Verification items for the finished model (mm, model axes). Coordinates: 2 decimals unless noted, no trailing zeros. Order: outer loops, then holes, each group sorted by start corner. A loop starts at its lowest first (then second) coordinate and runs counter-clockwise, first axis right, second up. Notation, with made-up numbers: M 36,-17.75 L 93,-17.75 A19 cw 93,10.25 Z; hole C 47,78 d8. An arc over 180 degrees is marked long. Return JSON: item names as keys, results as strings. Group by question number.
1. Material ranges on line 1 along Y through (x, z) = (27, 0.95); line 2 along X through (y, z) = (24.5, 1.35); line 3 along X through (y, z) = (26.5, 0.65), recorded low to high.
2. Section check C-C, the plane z = 1.95. Record the cut outline in (x, y), plus the area to 3 significant figures.
3. Mould release check, pull along X, two halves, no side actions. Record for faces 1 (the flat face through (44, 38, 0)), 2 (the cylindrical face through (55.532, 65.783, 1.479)), 3 (the flat face through (56, 34.748, 1)): +X half, -X half, draft (parallel to the pull), parting line (faces both ways), or undercut.
4. Gauge pin test, flat ends, axial feed: pin 1 (1.5 mm diameter, centred on x = 59, z = 2, fed in from +Y); pin 2 (1.5 mm diameter, centred on x = 55, z = 0.5, fed in from -Y); pin 3 (1.5 mm diameter, centred on x = 54, z = 1, fed in from -Y); pin 4 (1 mm diameter, centred on x = 15.5, y = 59, fed in from -Z). Record the tip position at first contact, or that the pin passes through.
5. Section check B-B, the plane x = 37.5. Record the cut outline in (y, z).
6. Section check D-D, the plane y = 16. Record the cut outline in (x, z), plus the area to 3 significant figures.
7. Section check A-A, the plane y = 37.5. Record the cut outline in (x, z).
```python
from build123d import *

# Parameters (mm, degrees)
F0_R     = 33.542405
F0_R_2   = 3
F1_DEPTH = 3


with BuildPart() as f1:
    # F0 (on Top) → F1 (new body)
    with BuildSketch(Plane.XY):
        with Locations((37.5, 37.5)):
            Circle(F0_R)
        with BuildLine():
            ThreePointArc((18.779471, 20.496946), (14.93532, 21.1058), (15.544173, 24.949951))
            Line((15.544173, 24.949951), (26.331132, 32.787135))
            ThreePointArc((26.331132, 32.787135), (30.175283, 32.178281), (29.566429, 28.33413))
            Line((29.566429, 28.33413), (18.779471, 20.496946))
        make_face(mode=Mode.SUBTRACT)
        with BuildLine():
            ThreePointArc((47.885903, 14.441486), (46.118941, 10.973627), (42.651082, 12.74059))
            Line((42.651082, 12.74059), (38.530831, 25.42142))
            ThreePointArc((38.530831, 25.42142), (40.297793, 28.889278), (43.765652, 27.122316))
            Line((43.765652, 27.122316), (47.885903, 14.441486))
        make_face(mode=Mode.SUBTRACT)
        with BuildLine():
            ThreePointArc((49.305957, 34.747892), (46.553848, 37.5), (49.305957, 40.252108))
            Line((49.305957, 40.252108), (62.639371, 40.252108))
            ThreePointArc((62.639371, 40.252108), (65.391479, 37.5), (62.639371, 34.747892))
            Line((62.639371, 34.747892), (49.305957, 34.747892))
        make_face(mode=Mode.SUBTRACT)
        with BuildLine():
            ThreePointArc((15.544173, 50.050049), (14.93532, 53.8942), (18.779471, 54.503054))
            Line((18.779471, 54.503054), (29.566429, 46.66587))
            ThreePointArc((29.566429, 46.66587), (30.175283, 42.821719), (26.331132, 42.212865))
            Line((26.331132, 42.212865), (15.544173, 50.050049))
        make_face(mode=Mode.SUBTRACT)
        with Locations((37.5, 37.5)):
            Circle(F0_R_2, mode=Mode.SUBTRACT)
        with BuildLine():
            ThreePointArc((42.651082, 62.25941), (46.118941, 64.026373), (47.885903, 60.558514))
            Line((47.885903, 60.558514), (43.765652, 47.877684))
            ThreePointArc((43.765652, 47.877684), (40.297793, 46.110722), (38.530831, 49.57858))
            Line((38.530831, 49.57858), (42.651082, 62.25941))
        make_face(mode=Mode.SUBTRACT)
    extrude(amount=F1_DEPTH)


solid = f1.part
```
Answers follow:
{
 "1": {"line 1": "5.64 to 26.47, 33.14 to 41.86, 48.53 to 69.36", "line 2": "6.58 to 15.06, 24.29 to 38.83, 44.62 to 68.42", "line 3": "5.81 to 17.68, 27.04 to 38.41, 43.97 to 69.19"},
 "2": {"outline": "C 37.5,37.5 d67.08; hole M 15.54,24.95 A2.75 ccw 18.78,20.5 L 29.57,28.33 A2.75 ccw 26.33,32.79 Z; hole M 15.54,50.05 L 26.33,42.21 A2.75 ccw 29.57,46.67 L 18.78,54.5 A2.75 ccw Z; hole C 37.5,37.5 d6; hole M 38.53,25.42 L 42.65,12.74 A2.75 ccw 47.89,14.44 L 43.77,27.12 A2.75 ccw Z; hole M 38.53,49.58 A2.75 ccw 43.77,47.88 L 47.89,60.56 A2.75 ccw 42.65,62.26 Z; hole M 49.31,34.75 L 62.64,34.75 A2.75 ccw 62.64,40.25 L 49.31,40.25 A2.75 ccw Z", "area": "3,020 mm^2"},
 "3": {"face 1": "draft", "face 2": "parting line", "face 3": "undercut"},
 "4": {"pin 1": "y = 63.85", "pin 2": "y = 8.44", "pin 3": "y = 7.89", "pin 4": "z = 0"},
 "5": {"outline": "M 3.96,0 L 34.5,0 L 34.5,3 L 3.96,3 Z; M 40.5,0 L 71.04,0 L 71.04,3 L 40.5,3 Z"},
 "6": {"outline": "M 11.75,0 L 41.59,0 L 41.59,3 L 11.75,3 Z; M 47.38,0 L 63.25,0 L 63.25,3 L 47.38,3 Z", "area": "137 mm^2"},
 "7": {"outline": "M 3.96,0 L 34.5,0 L 34.5,3 L 3.96,3 Z; M 40.5,0 L 46.55,0 L 46.55,3 L 40.5,3 Z; M 65.39,0 L 71.04,0 L 71.04,3 L 65.39,3 Z"}
}
